The model under review builds one solid part; all positions refer to its coordinate system, in mm. A direction names the side the tool comes from. Give positions to 0.01 mm unless a question says otherwise; leave off trailing zeros. Loops run counter-clockwise (first coordinate to the right, second up) from the corner with the lowest first, then second, coordinate; pieces in that order, holes last. Notation, with made-up numbers: M 28,51.25 L 49,51.25 A18 ccw 49,73.25 Z; hole C 55.5,36 d7. An arc over 180 degrees is marked long. One line per item, written item: value. Start each with the question number.
Q1. We need section A-A on z = 50.5. Write out the cut boundary in (x, y).
Q2. To check wall thickness, follow line 1 along X through (y, z) = (30.4, 55.6); line 2 along Z through (x, y) = (18, 39); line 3 along Y through (x, z) = (21, 35). State the ranges of each line that lie inside material, in increasing order. Write a range as from..to.
Q3. For pin 1 (2 mm diameter, centred on x = 12.5, z = 7.5, fed in from -Y); pin 2 (10.5 mm diameter, centred on x = 12.5, z = 29, fed in from +Y), all flat-tipped, find the tip position at first contact; note any pin that passes through.
Q4. Mouldability with a two-part tool opening along Y and no side actions: class faces 1 (the face through (12.761, 43.997, 56.521)), 2 (the face through (11.61, 0.99, 25)), 3 (the face through (13.441, 39.026, 1.521)) as released by +Y, released by -Y, zero draft, split by the parting line, or undercut.
Q5. For faces 4 (the face through (12, 19, 3)), 5 (the face through (12.272, 12.535, 1.521)), list the 3-axis set-ups (+Z, -Z, +X, -X, +Y, -Y) from which the entire face can be reached by the end or side of a thin tool; tool diameter is ignored.
Q6. We need section C-C on x = 12.5. Give the number of separate pieces and of enclosed holes in the cut face, plus the area to 3 significant figures.
Q7. We need section B-B on y = 20. Write out the cut boundary in (x, z), plus the area to 3 significant figures.
Q8. We need section D-D on y = 11.5. Write out the cut boundary in (x, z), plus the area to 3 significant figures.
Autodesk Inventor part; units mm, degrees
ref_plane "YZ Plane" through (0, 0, 0) normal (1, 0, 0) x (0, 1, 0)
ref_plane "XZ Plane" through (0, 0, 0) normal (0, 1, 0) x (-1, 0, 0)
ref_plane "XY Plane" through (0, 0, 0) normal (0, 0, 1) x (1, 0, 0)
sketch "Esboço1" plane through (0, 0, 0) normal (1, 0, 0) x (0, 1, 0)
  line L0 (0, 0) -> (50, 0)
  line L1 (50, 0) -> (50, 3)
  line L2 (50, 3) -> (2, 3)
  line L3 (2, 3) -> (2, 55)
  line L4 (2, 55) -> (50, 55)
  line L5 (50, 55) -> (50, 58)
  line L6 (50, 58) -> (0, 58)
  line L7 (0, 58) -> (0, 0)
  line L8 (2, 3) -> (0, 3)
  dimension "d84" = 52
  dimension "d85" = 3
  dimension "d86" = 3
  dimension "d87" = 3
  dimension "d90" = 2
extrude "Extrusão1" add sketch "Esboço1" along normal blind 25
sketch "Esboço2" plane through (0, 0, 58) normal (0, 0, 1) x (1, 0, 0)
  line L0 (0, 0) -> (25, 0)
  circle A0 centre (12.5, 10.8) radius 1.75
  circle A1 centre (12.5, 30.4) radius 4.1
  circle A2 centre (12.5, 23.25) radius 1.75
  line L1 (12.5, 30.4) -> (16.5, 30.4) construction
  line L2 (12.5, 30.4) -> (19.3, 30.4) construction
  circle A3 centre (7.6917, 25.5917) radius 1.25
  circle A4 centre (19.65, 30.4) radius 1.75
  circle A5 centre (12.5, 37.55) radius 1.75
  circle A6 centre (5.35, 30.4) radius 1.75
  circle A7 centre (17.3083, 25.5917) radius 1.25
  circle A8 centre (17.3083, 35.2083) radius 1.25
  circle A9 centre (7.6917, 35.2083) radius 1.25
  line L3 (0, 0) -> (25, 0)
  line L4 (29.4538, 30.4) -> (-4.4538, 30.4)
  line L5 (12.5, 39.3) -> (12.5, 0)
  line L6 (12.5, 39.3) -> (12.5, 44)
  line L7 (25, 2) -> (25, 50)
  line L8 (25, 50) -> (25, 30.4)
  arc A10 (25, 30.4) -> (0, 30.4) centre (12.5, 31.4555) ccw
  line L9 (0, 2) -> (0, 50)
  line L10 (0, 50) -> (25, 50)
  line L11 (0, 32.511) -> (0, 50)
  line L12 (0, 50) -> (25, 50)
  line L13 (25, 50) -> (25, 32.511)
  line L14 (0, 32.511) -> (0, 30.4)
  line L15 (25, 32.511) -> (25, 30.4)
  line L16 (25, 32.511) -> (25, 50)
  point P0 (25, 32.511)
  dimension "d11" = 3.5
  dimension "d14" = 8.2
  dimension "d26" = 3.5
  dimension "d42" = 2.5
  dimension "d50" = 1.3
  dimension "d53" = 360
  dimension "d59" = 360
  dimension "d61" = 10.8
  dimension "d62" = 39.3
  dimension "d63" = 4.7
extrude "Extrusão2" cut sketch "Esboço2" against normal through all contours A0 L5 | A1 L4 L5 | L5 L4 A1 | A2 L5 | L5 A2 | L5 A0 | A1 L5 L4 | L4 L5 A1 | L4 A6 | A6 L4 | L4 A4 | A4 L4 | L5 A5 | A5 L5 | A10 L9 L10 L7 | A3 | A7 | A8 | A9
sketch "Esboço4" plane through (0, 0, 0) normal (0, -1, 0) x (1, 0, 0)
  line L0 (0, 58) -> (25, 58)
  line L1 (14.25, 0) -> (10.75, 0)
  line L2 (25, 3) -> (25, 55)
  line L3 (0, 3) -> (0, 55)
  circle A0 centre (12.4993, 29.0025) radius 4.1
  circle A1 centre (12.4993, 21.6525) radius 1.75
  line L4 (12.4993, 29.0025) -> (16.4993, 29.0025) construction
  line L5 (12.4993, 29.0025) -> (19.2993, 29.0025) construction
  circle A2 centre (7.4434, 23.9467) radius 1.25
  circle A3 centre (19.8493, 29.0025) radius 1.75
  circle A4 centre (12.4993, 36.3525) radius 1.75
  circle A5 centre (5.1493, 29.0025) radius 1.75
  circle A6 centre (17.5551, 23.9467) radius 1.25
  circle A7 centre (17.5551, 34.0583) radius 1.25
  circle A8 centre (7.4434, 34.0583) radius 1.25
  circle A9 centre (12.5, 50.5) radius 1.75
  circle A10 centre (12.5, 7.5) radius 1.75
  line L6 (0, 0) -> (25, 0)
  line L7 (25, 58) -> (25, 0)
  line L8 (17.9, 3) -> (17.9, 0)
  line L9 (25, 58) -> (25, 0)
  line L10 (25, 29) -> (0, 29)
  line L11 (0, 58) -> (0, 0)
  line L12 (25, 58) -> (0, 58)
  line L13 (12.5, 58) -> (12.5, 0)
  point P0 (24.9565, 28.0304)
  dimension "d68" = 8.2
  dimension "d72" = 360
  dimension "d74" = 360
  dimension "d77" = 3.5
  dimension "d92" = 7.5
  dimension "d96" = 7.5
  dimension "d98" = 1.5
  dimension "d100" = 1.8
  dimension "d101" = 3.5
  dimension "d102" = 2.5
  dimension "d103" = 3.5
extrude "Extrusão3" cut sketch "Esboço4" against normal through all contours L13 A9 | A9 L13 | L10 A5 | A5 L10 | L13 A4 | A4 L13 | L10 A3 | A3 L10 | L10 L13 A0 | A0 L13 L10 | A0 L10 L13 | L13 L10 A0 | L13 A10 | A10 L13 | L13 A1 | A1 L13 | A2 | A6 | A7 | A8
properties part number "Medium FrameARRUMADO"
Solved:
1. outline: M 0,0 L 10.75,0 L 10.75,2 L 0,2 Z; M 14.25,0 L 25,0 L 25,2 L 14.25,2 Z
2. line 1: 0..3.6, 7.1..8.4, 16.6..17.9, 21.4..25
2. line 2: 0..3, 55..58
2. line 3: 0..2
3. pin 1: through
3. pin 2: y = 2
4. face 1: released by +Y
4. face 2: zero draft
4. face 3: undercut
5. face 4: +X, -X, +Y
5. face 5: +Z, -Z
6. separate pieces: 14
6. enclosed holes: 0
6. area: 211 mm2
7. outline: M 0,0 L 25,0 L 25,3 L 0,3 Z; M 0,55 L 25,55 L 25,58 L 0,58 Z
7. area: 150 mm2
8. outline: M 0,0 L 10.9,0 L 10.9,3 L 0,3 Z; M 0,55 L 10.9,55 L 10.9,58 L 0,58 Z; M 14.1,0 L 25,0 L 25,3 L 14.1,3 Z; M 14.1,55 L 25,55 L 25,58 L 14.1,58 Z
8. area: 131 mm2
